from build123d import *

# Parameters (mm, degrees)
SKETCH1_W           = 39
SKETCH1_H           = 23.712741858
BOSS_EXTRUDE1_DEPTH = 2
SKETCH9_R           = 4.05
CUT_EXTRUDE6_DEPTH  = 5
SKETCH10_R          = 1.25
BOSS_EXTRUDE5_DEPTH = 5.5
SKETCH11_R          = 2.5
CUT_EXTRUDE7_DEPTH  = 5
BOSS_EXTRUDE6_START = -5.5
SKETCH12_R          = 2.5
BOSS_EXTRUDE6_DEPTH = 5.5
BOSS_EXTRUDE7_DEPTH = 28


with BuildPart() as part:
    # Sketch1 → Boss-Extrude1 (new body)
    with BuildSketch(Plane.XY):
        with Locations((0, -11)):
            Rectangle(SKETCH1_W, SKETCH1_H)
        with BuildLine():
            ThreePointArc((1.25, -19), (0, -17.75), (-1.25, -19))
            ThreePointArc((-1.25, -19), (0, -20.25), (1.25, -19))
        make_face(mode=Mode.SUBTRACT)
        with BuildLine():
            ThreePointArc((-6.75, -11), (-8, -9.75), (-9.25, -11))
            ThreePointArc((-9.25, -11), (-8, -12.25), (-6.75, -11))
        make_face(mode=Mode.SUBTRACT)
        with BuildLine():
            ThreePointArc((1.25, -3), (0, -1.75), (-1.25, -3))
            ThreePointArc((-1.25, -3), (0, -4.25), (1.25, -3))
        make_face(mode=Mode.SUBTRACT)
        with BuildLine():
            ThreePointArc((9.25, -11), (8, -9.75), (6.75, -11))
            ThreePointArc((6.75, -11), (8, -12.25), (9.25, -11))
        make_face(mode=Mode.SUBTRACT)
    extrude(amount=BOSS_EXTRUDE1_DEPTH)

    # Sketch9 → Cut-Extrude6 (cut)
    with BuildSketch(Plane.XY.offset(2)):
        with Locations((0, -11)):
            Circle(SKETCH9_R)
    extrude(amount=-CUT_EXTRUDE6_DEPTH, mode=Mode.SUBTRACT)

    # Sketch10 → Boss-Extrude5 (add)
    # profile 1 of 2: a face of its own
    with BuildSketch(Plane.ZY.offset(19.5)):
        with BuildLine():
            Line((4.2, 3.5), (8.5, 3.5))
            Line((8.5, 3.5), (8.5, 0.5))
            ThreePointArc((8.5, 0.5), (7.474873734, -1.974873734), (5, -3))
            Line((5, -3), (2, -3))
            Line((2, -3), (2, 0.856370929))
            Line((2, 0.856370929), (0, 0.856370929))
            Line((0, 0.856370929), (0, 3.5))
            Line((0, 3.5), (4.2, 3.5))
        make_face()
        with Locations((5.25, 0.25)):
            Circle(SKETCH10_R, mode=Mode.SUBTRACT)
    # profile 2 of 2: a face of its own
    with BuildSketch(Plane.ZY.offset(19.5)):
        with BuildLine():
            Line((5, -19), (2, -19))
            Line((2, -19), (2, -22.856370929))
            Line((2, -22.856370929), (0, -22.856370929))
            Line((0, -22.856370929), (0, -25.5))
            Line((0, -25.5), (4.2, -25.5))
            Line((4.2, -25.5), (8.5, -25.5))
            Line((8.5, -25.5), (8.5, -22.5))
            ThreePointArc((8.5, -22.5), (7.474873734, -20.025126266), (5, -19))
        make_face()
        with Locations((5.25, -22.25)):
            Circle(SKETCH10_R, mode=Mode.SUBTRACT)
    extrude(amount=-BOSS_EXTRUDE5_DEPTH)

    # Sketch11 → Cut-Extrude7 (cut)
    with BuildSketch(Plane.ZY.offset(19.5)):
        with Locations((5.25, 0.25)):
            Circle(SKETCH11_R)
        with Locations(Location((5.25, -22.25, 0), (0, 0, 180))):
            Circle(SKETCH11_R)
    extrude(amount=-CUT_EXTRUDE7_DEPTH, mode=Mode.SUBTRACT)

    # Sketch12 → Boss-Extrude6 (add)
    with BuildSketch(Plane(origin=(19.5, 0, 0), x_dir=(0, 0, -1), z_dir=(1, 0, 0)).offset(BOSS_EXTRUDE6_START)):
        with BuildLine():
            ThreePointArc((-8.5, 0.5), (-7.474873734, -1.974873734), (-5, -3))
            Line((-5, -3), (-2, -3))
            Line((-2, -3), (-2, -19))
            Line((-2, -19), (-5, -19))
            ThreePointArc((-5, -19), (-7.474873734, -20.025126266), (-8.5, -22.5))
            Line((-8.5, -22.5), (-8.5, -25.5))
            Line((-8.5, -25.5), (0, -25.5))
            Line((0, -25.5), (0, 3.5))
            Line((0, 3.5), (-8.5, 3.5))
            Line((-8.5, 3.5), (-8.5, 0.5))
        make_face()
        with Locations((-5.25, -22.25)):
            Circle(SKETCH12_R, mode=Mode.SUBTRACT)
        with Locations(Location((-5.25, 0.25, 0), (0, 0, 180))):
            Circle(SKETCH12_R, mode=Mode.SUBTRACT)
    extrude(amount=BOSS_EXTRUDE6_DEPTH)

    # Sketch13 → Boss-Extrude7 (add)
    with BuildSketch(Plane.ZY.offset(-14)):
        Polygon((0, 3.5), (4.2, 3.5), (2, 1.3), (2, 0.856370929), (0, 0.856370929), align=None)
        Polygon((2, -22.856370929), (0, -22.856370929), (0, -25.5), (4.2, -25.5), (2, -23.3), align=None)
    extrude(amount=BOSS_EXTRUDE7_DEPTH)


solid = part.part
Build history of the part. All positions in model axes, mm. A direction names the side the tool comes from. Round coordinates to 2 decimals unless told otherwise and drop trailing zeros. Write each loop counter-clockwise with the first axis right and the second up, starting at its lowest first coordinate (ties: lowest second). Pieces come first, ordered by that corner, then holes. Notation, with made-up numbers: M 63.25,61 L 98.25,61 A10 cw 98.25,71 Z; hole C 9.5,34.25 d5. An arc over 180 degrees is marked long. Answer as a JSON object with one key per item and string values. Group by question number.
(1) Cut at D-D (x = 0). Give the cut face in (y, z).
(2) Cut at A-A (x = -8). Give the cut face in (y, z), and give its area (3 significant figures).
(3) Flat gauge pins, fed straight in: pin 1 (1.5 mm diameter, centred on x = 12.5, y = -15.5, fed in from +Z); pin 2 (2 mm diameter, centred on x = -8, y = -11, fed in from +Z); pin 3 (2.5 mm diameter, centred on y = -21.5, z = 6, fed in from -X); pin 4 (3 mm diameter, centred on y = 0.25, z = 5.25, fed in from +X). Where does each tip first touch, or does it go through?
(4) Which spindle directions (+Z, -Z, +X, -X, +Y, -Y) get a long thin tool onto all of the face, cutting with end or side? Do faces 1 (the cylindrical face through (0.27, -17.78, 0.99)), 2 (the flat face through (0, -25.5, 3)), 3 (the flat face through (-14.5, -21, 4)), 4 (the cylindrical face through (16.71, -20, 7.45)), 5 (the flat face through (0.2, 2.4, 3.1)). Say none if no direction does.
(5) Drill centre lines: L1, parallel to Y at x = -16.1, z = 5.25; L2, parallel to Y at x = -14.25, z = 5.25; L3, parallel to X at y = -19, z = 0.7. Where is each one in solid material? Low to high.
(6) Cut at B-B (z = 0.5). Give the cut face in (x, y).
(7) Cut at C-C (y = -11). Give the cut face in (x, z).
(8) Mould opens along Z. For faces 6 (the cylindrical face through (-16.79, -20.05, 7.5)), 7 (the flat face through (5, -11, 0)), 8 (the cylindrical face through (-14.25, -23.47, 4.98)), 9 (the cylindrical face through (8.921, -11.845, 0.986)) say: pulls with the +Z half, pulls with the -Z half, needs draft (parallel to the pull), parting line crosses it, or undercut.
Responses:
{
 "1": {"outline": "M -25.5,0 L -20.25,0 L -20.25,2 L -23.3,2 L -25.5,4.2 Z; M -17.75,0 L -15.05,0 L -15.05,2 L -17.75,2 Z; M -6.95,0 L -4.25,0 L -4.25,2 L -6.95,2 Z; M -1.75,0 L 3.5,0 L 3.5,4.2 L 1.3,2 L -1.75,2 Z"},
 "2": {"outline": "M -25.5,0 L -12.25,0 L -12.25,2 L -23.3,2 L -25.5,4.2 Z; M -9.75,0 L 3.5,0 L 3.5,4.2 L 1.3,2 L -9.75,2 Z", "area": "57.8 mm2"},
 "3": {"pin 1": "stops at z = 2", "pin 2": "passes through", "pin 3": "stops at x = -14.5", "pin 4": "stops at x = -14"},
 "4": {"face 1": "+Z, -Z", "face 2": "+Z, -Z, +X, -X, -Y", "face 3": "-X", "face 4": "+Z, +X, -X", "face 5": "+Z"},
 "5": {"L1": "y = -25.5 to -24.75, -19.75 to -19.01, -2.99 to -2.25, 2.75 to 3.5", "L2": "y = -25.5 to -23.5, -21 to -19.01, -2.99 to -1, 1.5 to 3.5", "L3": "x = -19.5 to -1.25, 1.25 to 19.5"},
 "6": {"outline": "M -19.5,-25.5 L 19.5,-25.5 L 19.5,3.5 L -19.5,3.5 Z; hole C -8,-11 d2.5; hole C 0,-11 d8.1; hole C 0,-19 d2.5; hole C 0,-3 d2.5; hole C 8,-11 d2.5"},
 "7": {"outline": "M -19.5,0 L -9.25,0 L -9.25,2 L -19.5,2 Z; M -6.75,0 L -4.05,0 L -4.05,2 L -6.75,2 Z; M 4.05,0 L 6.75,0 L 6.75,2 L 4.05,2 Z; M 9.25,0 L 19.5,0 L 19.5,2 L 9.25,2 Z"},
 "8": {"face 6": "pulls with the +Z half", "face 7": "pulls with the -Z half", "face 8": "undercut", "face 9": "needs draft"}
}
